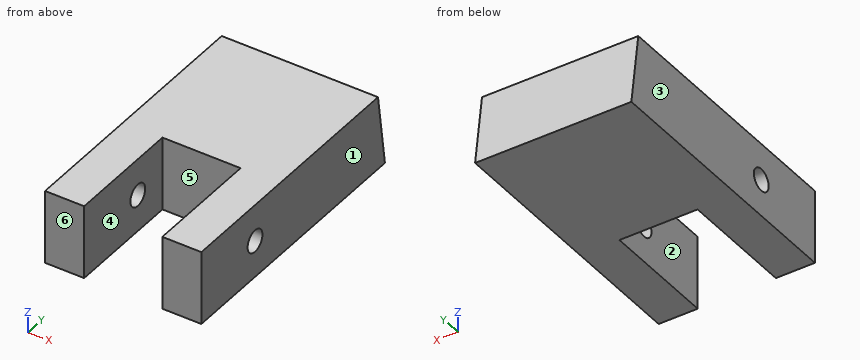
from build123d import *

# Parameters (mm, degrees)
BOSS_EXTRUDE1_DEPTH  = 25.4
SKETCH2_W            = 12.7
SKETCH2_H            = 19.05
CUT_EXTRUDE1_DEPTH   = 53.76066686
M3_CLEARANCE_HOLE1_D = 3.6


with BuildPart() as part:
    # Sketch1 → Boss-Extrude1 (new body)
    with BuildSketch(Plane(origin=(0, 0, 0), x_dir=(0, 0, -1), z_dir=(1, 0, 0))):
        Polygon((0, 0), (11.9888, 0), (11.9888, 44.663146352), (0, 42.978230393), align=None)
    extrude(amount=BOSS_EXTRUDE1_DEPTH)

    # Sketch2 → Cut-Extrude1 (cut, through all)
    with BuildSketch(Plane.XY):
        with Locations((12.7, 9.525)):
            Rectangle(SKETCH2_W, SKETCH2_H)
    extrude(amount=-CUT_EXTRUDE1_DEPTH, mode=Mode.SUBTRACT)

    # M3 Clearance Hole1 (through all)
    with Locations(Plane(origin=(25.4, 0, 0), x_dir=(0, 0, -1), z_dir=(1, 0, 0))):
        with Locations((5.9944, 13.0556)):
            Hole(M3_CLEARANCE_HOLE1_D / 2)


solid = part.part
The model under review builds one solid part; all positions refer to its coordinate system, in mm. Face numbers are marked on the shaded views. A direction names the side the tool comes from. Coordinates: 2 decimals unless noted, no trailing zeros. Write each loop counter-clockwise with the first axis right and the second up, starting at its lowest first coordinate (ties: lowest second). Pieces come first, ordered by that corner, then holes. Notation, with made-up numbers: (58.5, 1.5) - (76.5, 1.5) arc R9 cw to (76.5, 8.5) - close; hole circle Ø7 at (3, -2). An arc over 180 degrees is marked (long way). Answer as a JSON object with one key per item and string values. Group by question number.
1. Clearance check with flat-ended pins moving along their axes: pin 1 Ø6 at (x, z) = (10, -4.5) entering from +Y; pin 2 Ø3 at (x, z) = (5, -6.5) entering from +Y; pin 3 Ø3.5 at (x, z) = (11.5, -6) entering from -Y. State where each tip first meets the part, or that it passes through.
2. To check wall thickness, follow probe 1 along X at (y, z) = (16.5, -1.5); probe 2 along Z at (x, y) = (23, 11.5). State the ranges of each line that lie inside material, in increasing order.
3. Add section D-D (z = -9.25). Give the boundary of the cut face in (x, y), plus the area to 3 significant figures.
4. Add section B-B (z = -7). Give the boundary of the cut face in (x, y), plus the area to 3 significant figures.
5. Mouldability with a two-part tool opening along X and no side actions: class the marked faces 3, 4, 5 and 6 as pulls with the +X half, pulls with the -X half, needs draft (parallel to the pull), parting line crosses it, or undercut.
6. Add section A-A (y = 9.5). Give the boundary of the cut face in (x, z), plus the area to 3 significant figures.
7. Add section C-C (x = 10.5). Give the boundary of the cut face in (y, z).
8. Machinability: for the marked faces 1 and 2, which of the approach directions +Z, -Z, +X, -X, +Y, -Y give a long, thin tool a straight path to every point of the face, cutting with its end or side? Answer none if there is none.
Findings:
{
 "1": {"pin 1": "y = 44.03", "pin 2": "y = 44.1", "pin 3": "y = 19.05"},
 "2": {"probe 1": "0 to 6.35, 19.05 to 25.4", "probe 2": "-11.99 to -6.9, -5.09 to 0"},
 "3": {"outline": "(0, 0) - (6.35, 0) - (6.35, 19.05) - (19.05, 19.05) - (19.05, 0) - (25.4, 0) - (25.4, 44.28) - (0, 44.28) - close", "area": "883 mm²"},
 "4": {"outline": "(0, 0) - (6.35, 0) - (6.35, 11.56) - (0, 11.56) - close; (0, 14.55) - (6.35, 14.55) - (6.35, 19.05) - (19.05, 19.05) - (19.05, 14.55) - (25.4, 14.55) - (25.4, 43.96) - (0, 43.96) - close; (19.05, 0) - (25.4, 0) - (25.4, 11.56) - (19.05, 11.56) - close", "area": "837 mm²"},
 "5": {"face 3": "pulls with the -X half", "face 4": "undercut", "face 5": "undercut", "face 6": "needs draft"},
 "6": {"outline": "(0, -11.99) - (6.35, -11.99) - (6.35, 0) - (0, 0) - close; (19.05, -11.99) - (25.4, -11.99) - (25.4, 0) - (19.05, 0) - close", "area": "152 mm²"},
 "7": {"outline": "(19.05, -11.99) - (44.66, -11.99) - (42.98, 0) - (19.05, 0) - close"},
 "8": {"face 1": "+Z, -Z, +X, +Y, -Y", "face 2": "+Z, -Z, -Y"}
}
